from build123d import *

# Parameters (mm, degrees)
SKETCH1_R               = 150
SKETCH1_R_2             = 97.5
SKETCH1_R_3             = 11.75
BOSS_EXTRUDE1_DEPTH     = 30
SKETCH1_3_R             = 97.5
SKETCH1_3_R_2           = 40.15
SKETCH1_3_R_3           = 17.5
SKETCH1_3_R_4           = 6
BOSS_EXTRUDE2_DEPTH     = 38
SKETCH1_4_R             = 40.15
SKETCH1_4_R_2           = 35
BOSS_EXTRUDE3_DEPTH     = 40
BOSS_EXTRUDE4_START     = 38
SKETCH1_5_R             = 17.5
SKETCH1_5_R_2           = 11.5
BOSS_EXTRUDE4_DEPTH     = 14
SKETCH2_R               = 43.5
CUT_EXTRUDE1_DEPTH      = 1
CUT_EXTRUDE1_DEPTH_BACK = 5


with BuildPart() as part:
    # Sketch1 → Boss-Extrude1 (new body)
    with BuildSketch(Plane(origin=(0, 0, 0), x_dir=(1, 0, 0), z_dir=(0, 1, 0))):
        Circle(SKETCH1_R)
        Circle(SKETCH1_R_2, mode=Mode.SUBTRACT)
        with Locations((-89.802561211, -89.802561211)):
            Circle(SKETCH1_R_3, mode=Mode.SUBTRACT)
        with Locations((89.802561211, -89.802561211)):
            Circle(SKETCH1_R_3, mode=Mode.SUBTRACT)
        with Locations((89.802561211, 89.802561211)):
            Circle(SKETCH1_R_3, mode=Mode.SUBTRACT)
        with Locations((-89.802561211, 89.802561211)):
            Circle(SKETCH1_R_3, mode=Mode.SUBTRACT)
    extrude(amount=BOSS_EXTRUDE1_DEPTH)

    # Sketch1<3> → Boss-Extrude2 (add)
    with BuildSketch(Plane(origin=(0, 0, 0), x_dir=(1, 0, 0), z_dir=(0, 1, 0))):
        Circle(SKETCH1_3_R)
        Circle(SKETCH1_3_R_2, mode=Mode.SUBTRACT)
        with Locations((-28.338059011, 69.440293861)):
            Circle(SKETCH1_3_R_3, mode=Mode.SUBTRACT)
        with Locations((-69.440293861, -28.338059011)):
            Circle(SKETCH1_3_R_3, mode=Mode.SUBTRACT)
        with Locations((28.338059011, -69.440293861)):
            Circle(SKETCH1_3_R_3, mode=Mode.SUBTRACT)
        with Locations((69.440293861, 28.338059011)):
            Circle(SKETCH1_3_R_3, mode=Mode.SUBTRACT)
        with Locations((-60, 60)):
            Circle(SKETCH1_3_R_4, mode=Mode.SUBTRACT)
    extrude(amount=BOSS_EXTRUDE2_DEPTH)

    # Sketch1<4> → Boss-Extrude3 (add)
    with BuildSketch(Plane(origin=(0, 0, 0), x_dir=(1, 0, 0), z_dir=(0, 1, 0))):
        Circle(SKETCH1_4_R)
        Circle(SKETCH1_4_R_2, mode=Mode.SUBTRACT)
    extrude(amount=BOSS_EXTRUDE3_DEPTH)

    # Sketch1<5> → Boss-Extrude4 (add)
    with BuildSketch(Plane(origin=(0, 0, 0), x_dir=(1, 0, 0), z_dir=(0, 1, 0)).offset(BOSS_EXTRUDE4_START)):
        with Locations((-28.338059011, 69.440293861)):
            Circle(SKETCH1_5_R)
        with Locations((-28.338059011, 69.440293861)):
            Circle(SKETCH1_5_R_2, mode=Mode.SUBTRACT)
        with Locations((69.440293861, 28.338059011)):
            Circle(SKETCH1_5_R)
        with Locations((69.440293861, 28.338059011)):
            Circle(SKETCH1_5_R_2, mode=Mode.SUBTRACT)
        with Locations((28.338059011, -69.440293861)):
            Circle(SKETCH1_5_R)
        with Locations((28.338059011, -69.440293861)):
            Circle(SKETCH1_5_R_2, mode=Mode.SUBTRACT)
        with Locations((-69.440293861, -28.338059011)):
            Circle(SKETCH1_5_R)
        with Locations((-69.440293861, -28.338059011)):
            Circle(SKETCH1_5_R_2, mode=Mode.SUBTRACT)
    extrude(amount=-BOSS_EXTRUDE4_DEPTH)

    # Sketch2 → Cut-Extrude1 (cut, two sides)
    with BuildSketch(Plane.XZ) as cut_extrude1_sk:
        Circle(SKETCH2_R)
    extrude(amount=CUT_EXTRUDE1_DEPTH, mode=Mode.SUBTRACT)
    extrude(cut_extrude1_sk.sketch, amount=-CUT_EXTRUDE1_DEPTH_BACK, mode=Mode.SUBTRACT)


solid = part.part
Geometry: final body of the model. Coordinates: model frame, mm. A direction names the side the tool comes from. Give positions to 0.01 mm unless a question says otherwise; leave off trailing zeros. Write each loop counter-clockwise with the first axis right and the second up, starting at its lowest first coordinate (ties: lowest second). Pieces come first, ordered by that corner, then holes. Notation, with made-up numbers: (1, 21.5) -> (22, 21.5) arc R23 cw to (22, 43.5) -> close; hole circle Ø11 at (76, -12). An arc over 180 degrees is marked (long way). Answer in a Markdown table with one row per item.
(1) Set-up query: faces 1 (the cylindrical face through (-78.95, 14.79, -85.3)), 2 (the flat face through (98, 30, -2)), 3 (the flat face through (73, 24, -17)). Return all of +Z, -Z, +X, -X, +Y, -Y with unobstructed straight access to the full face (end or side cutting, diameter ignored); none if empty.
Answers below:
| item | result |
|---|---|
| face 1 | +Y, -Y |
| face 2 | +Y |
| face 3 | -Y |
(2) Pin query (flat end, axial travel): pin 1 (3 mm diameter, centred on y = 15.5, z = -30.5, fed in from -X); pin 2 (18.5 mm diameter, centred on x = 69.44, z = -28.34, fed in from +Y); pin 3 (1.5 mm diameter, centred on x = 16, y = 34, fed in from +Z); pin 4 (2 mm diameter, centred on x = 39.5, y = 13, fed in from +Z) (3 decimals). Return the tip coordinate at first contact, or that it passes through.
Answers below:
| item | result |
|---|---|
| pin 1 | x = -147.17 |
| pin 2 | through |
| pin 3 | z = 96.3 |
| pin 4 | z = 144.975 |
(3) Draft query along X for faces 4 (the cylindrical face through (-19.527, 14.79, -148.724)), 5 (the flat face through (31, 0, 31)), 6 (the cylindrical face through (-84.381, 14.79, 100.227)). Return one class per face: +X half, -X half, draft (parallel to the pull), parting line (faces both ways), or undercut.
Answers below:
| item | result |
|---|---|
| face 4 | parting line |
| face 5 | draft |
| face 6 | undercut |
(4) Ray query, line 1 along Z through (x, y) = (31, 17.5); line 2 along X through (y, z) = (22, -60); line 3 along X through (y, z) = (24, 0). Return the intervals inside material, ascending. Write a range as [from, to].
Answers below:
| item | result |
|---|---|
| line 1 | [-146.76, -16.25], [16.25, 52.14], [86.74, 146.76] |
| line 2 | [-137.48, -66], [-54, -43.07], [-13.6, 137.48] |
| line 3 | [-150, -35], [35, 150] |
(5) Section query A-A on x = 0. Return loops of the section in (y, z).
Answers below:
| item | result |
|---|---|
| outline | (0, -150) -> (30, -150) -> (30, -97.5) -> (38, -97.5) -> (38, -40.15) -> (40, -40.15) -> (40, -35) -> (5, -35) -> (5, -43.5) -> (0, -43.5) -> close; (0, 43.5) -> (5, 43.5) -> (5, 35) -> (40, 35) -> (40, 40.15) -> (38, 40.15) -> (38, 97.5) -> (30, 97.5) -> (30, 150) -> (0, 150) -> close |
(6) Section query B-B on z = 0. Return loops of the section in (x, y), then the cut area to 3 significant figures.
Answers below:
| item | result |
|---|---|
| outline | (-150, 0) -> (-43.5, 0) -> (-43.5, 5) -> (-35, 5) -> (-35, 40) -> (-40.15, 40) -> (-40.15, 38) -> (-97.5, 38) -> (-97.5, 30) -> (-150, 30) -> close; (35, 5) -> (43.5, 5) -> (43.5, 0) -> (150, 0) -> (150, 30) -> (97.5, 30) -> (97.5, 38) -> (40.15, 38) -> (40.15, 40) -> (35, 40) -> close |
| area | 7,840 mm^2 |
(7) Section query C-C on y = 16. State how many separate pieces and enclosed holes the cut face has, then the cut area to 3 significant figures.
Answers below:
| item | result |
|---|---|
| separate pieces | 1 |
| enclosed holes | 10 |
| area | 61,100 mm^2 |
